Read the model definition and answer for the solid it produces. Units are mm, in the model's axes. Give positions to 0.01 mm unless a question says otherwise; leave off trailing zeros. Loops run counter-clockwise (first coordinate to the right, second up) from the corner with the lowest first, then second, coordinate; pieces in that order, holes last. Notation, with made-up numbers: (-25.5, 38) - (12.5, 38) arc R9 ccw to (12.5, 50) - close; hole circle Ø11 at (14.25, -33.75). An arc over 180 degrees is marked (long way). Write each question's results on one line, items separated by ' | '. Start each with the question number.
Q1. Determine the mould class of faces 1 (the flat face through (-26, -37.945, 26)), 2 (the conical face through (-27.162, -13.157, -8.554)), 3 (the cylindrical face through (47.032, 1.786, 36.063)) for opening direction X: +X half, -X half, draft (parallel to the pull), parting line (faces both ways), or undercut.
Q2. The part is cut by section B-B, the plane x = 0. Write down the section's boundary in (y, z), plus the area to 3 significant figures.
Q3. Given pin 1 (1 mm diameter, centred on x = -43.5, y = -9.5, fed in from +Z); pin 2 (1.5 mm diameter, centred on y = -30, z = 11, fed in from -X); pin 3 (2 mm diameter, centred on x = -18, y = -22.5, fed in from +Z), each flat-ended and moving along its own axis, determine where each tip first touches the part or whether it passes through.
Q4. The part is cut by section D-D, the plane y = 26.5. Write down the section's boundary in (x, z).
Q5. The part is cut by section C-C, the plane y = 10. Write down the section's boundary in (x, z), plus the area to 3 significant figures.
Q6. The part is cut by section A-A, the plane z = 0. Write down the section's boundary in (x, y).
Q7. Find the intervals of material crossed by line 1 (Z direction, x = 4, y = 27.5); line 2 (Z direction, x = 22, y = -13); line 3 (X direction, y = 22, z = 13), in increasing order. Write a range as from..to.
Autodesk Inventor part; units mm, degrees
ref_plane "YZ Plane" through (0, 0, 0) normal (1, 0, 0) x (0, 1, 0)
ref_plane "XZ Plane" through (0, 0, 0) normal (0, 1, 0) x (-1, 0, 0)
ref_plane "XY Plane" through (0, 0, 0) normal (0, 0, 1) x (1, 0, 0)
sketch "Sketch1" plane through (0, 0, 0) normal (0, 0, 1) x (1, 0, 0)
  arc A0 (-25.8327, -3.287) -> (-25.4, 0) centre (-38.1, 0) ccw
  line L0 (-59.2667, 42.6459) -> (-60.6149, 42.6459)
  line L1 (-59.2667, 42.6459) -> (0, 42.6459) construction
  line L2 (-41.4694, -37.9453) -> (-35.1194, -37.9453)
  line L3 (-80.7, -43.0791) -> (-21.9625, -43.0791) construction
  line L4 (-87.05, -219.9038) -> (-83.875, -219.9038)
  line L5 (0, 42.6459) -> (0, 0)
  line L6 (-87.8501, 55.3459) -> (-18.3062, 55.3459) construction
  line L7 (-87.8501, 55.3459) -> (-14.7047, 55.3459) construction
  line L8 (-87.8501, 55.3459) -> (-52.22, 55.3459) construction
  arc A1 (-25.4, 0) -> (-55.5582, 40.2879) centre (-67.3891, 0) ccw
  line L9 (-59.2667, 42.6459) -> (-59.2667, -37.9453)
  line L10 (-59.2667, 42.6459) -> (21.3245, 42.6459) construction
  line L11 (-59.2667, -37.9453) -> (-41.4694, -37.9453)
  line L12 (-55.5582, 40.2879) -> (-59.2667, 42.6459)
  line L13 (-35.1194, -37.9453) -> (-25.8327, -3.287)
  dimension "d56" = 25.4
  dimension "d60" = 12.7
  dimension "d61" = 12.7
  dimension "d62" = 59.2667
  dimension "d63" = 6.35
  dimension "d77" = 3.175
  dimension "d84" = 41.9891
  dimension "d85" = 32.2919
  dimension "d86" = 90
  dimension "d87" = 80.5912
revolve "Revolution1" add sketch "Sketch1" angle 360 about axis through (0, 42.6459, 0) along (0, -1, 0)
properties part number "Graphite" material "GFRC"
Check sheet entries:
1) face 1: draft | face 2: undercut | face 3: parting line
2) outline: (-37.95, -59.27) - (42.65, -59.27) - (40.29, -55.56) arc R41.99 ccw to (0, -25.4) arc R12.7 ccw to (-3.29, -25.83) - (-37.95, -35.12) - close; (-37.95, 35.12) - (-3.29, 25.83) arc R12.7 ccw to (0, 25.4) arc R41.99 ccw to (40.29, 55.56) - (42.65, 59.27) - (-37.95, 59.27) - close | area: 4,310 mm^2
3) pin 1: stops at z = 40.79 | pin 2: stops at x = -58.37 | pin 3: stops at z = 56.78
4) outline: circle Ø118.53 at (0, 0); hole circle Ø69.64 at (0, 0)
5) outline: circle Ø118.53 at (0, 0); hole circle Ø53.22 at (0, 0) | area: 8,810 mm^2
6) outline: (-59.27, -37.95) - (-35.12, -37.95) - (-25.83, -3.29) arc R12.7 ccw to (-25.4, 0) arc R41.99 ccw to (-55.56, 40.29) - (-59.27, 42.65) - close; (25.4, 0) arc R12.7 ccw to (25.83, -3.29) - (35.12, -37.95) - (59.27, -37.95) - (59.27, 42.65) - (55.56, 40.29) arc R41.99 ccw to start
7) line 1: z = -59.13..-35.43, 35.43..59.13 | line 2: z = -55.03..-18.02, 18.02..55.03 | line 3: x = -57.82..-28.83, 28.83..57.82
